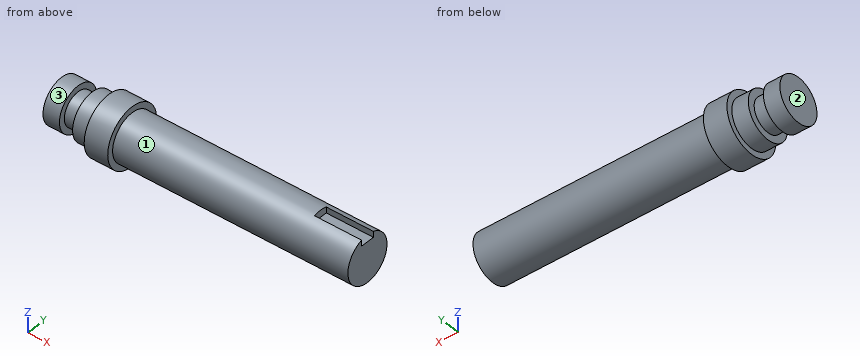
```python
from build123d import *

# Parameters (mm, degrees)
CUT_EXTRUDE1_DEPTH = 20


with BuildPart() as part:
    # Sketch1 → Revolve1 (revolve)
    with BuildSketch(Plane.XY, mode=Mode.PRIVATE) as revolve1_sk:
        Polygon((0, 0), (0, 9.5), (7, 9.5), (7, 7), (13, 7), (13, 10), (20, 10), (20, 12.5), (30, 12.5), (30, 10), (130, 10), (130, 0), align=None)
    revolve(revolve1_sk.sketch.rotate(Axis((130, 0, 0), (-1, 0, 0)), 90), axis=Axis((130, 0, 0), (-1, 0, 0)))

    # Sketch2 → Cut-Extrude1 (cut)
    with BuildSketch(Plane(origin=(130, 0, 0), x_dir=(0, 0, -1), z_dir=(1, 0, 0))):
        with BuildLine():
            Line((-9.539392014, 3), (-7.039392014, 3))
            Line((-7.039392014, 3), (-7.039392014, -3))
            Line((-7.039392014, -3), (-9.539392014, -3))
            ThreePointArc((-9.539392014, -3), (-10, 0), (-9.539392014, 3))
        make_face()
    extrude(amount=-CUT_EXTRUDE1_DEPTH, mode=Mode.SUBTRACT)


solid = part.part
```
The listing builds one solid part. Answer for the finished solid, in the listing's coordinates (mm). Face numbers are marked on the shaded views. A direction names the side the tool comes from. Round coordinates to 2 decimals unless told otherwise and drop trailing zeros. Loops run counter-clockwise (first coordinate to the right, second up) from the corner with the lowest first, then second, coordinate; pieces in that order, holes last.
Q1. Which of the six approach directions +Z, -Z, +X, -X, +Y, -Y give full straight-line access (tool end or side, diameter ignored) to the marked faces 1, 2 and 3?
Q2. Section C-C, the plane x = 56 is taken. Determine the outline of the cut face in (y, z), then the cut area to 3 significant figures.
Q3. Section A-A, the plane y = 0 is taken. Determine the outline of the cut face in (x, z).
Q4. Find the intervals of material crossed by line 1 (X direction, y = -2.5, z = 8.5); line 2 (X direction, y = -8.5, z = 1.5); line 3 (X direction, y = -11.5, z = 2.75), in increasing order.
Q5. Section B-B, the plane z = 0 is taken. Determine the outline of the cut face in (x, y).
Q6. Given pin 1 Ø6.5 at (x, y) = (124.5, -0.5) entering from +Z; pin 2 Ø6 at (x, z) = (31, -5.5) entering from -Y; pin 3 Ø6 at (x, y) = (74.5, -1) entering from -Z, each flat-ended and moving along its own axis, determine where each tip first touches the part or whether it passes through.
Completed:
1. face 1: +X
1. face 2: +Z, -Z, -X, +Y, -Y
1. face 3: -X
2. outline: circle Ø20 at (0, 0)
2. area: 314 mm2
3. outline: (0, -9.5) - (7, -9.5) - (7, -7) - (13, -7) - (13, -10) - (20, -10) - (20, -12.5) - (30, -12.5) - (30, -10) - (130, -10) - (130, 7.04) - (110, 7.04) - (110, 10) - (30, 10) - (30, 12.5) - (20, 12.5) - (20, 10) - (13, 10) - (13, 7) - (7, 7) - (7, 9.5) - (0, 9.5) - close
4. line 1: x = 0 to 7, 13 to 110
4. line 2: x = 0 to 7, 13 to 130
4. line 3: x = 20 to 30
5. outline: (0, -9.5) - (7, -9.5) - (7, -7) - (13, -7) - (13, -10) - (20, -10) - (20, -12.5) - (30, -12.5) - (30, -10) - (130, -10) - (130, 10) - (30, 10) - (30, 12.5) - (20, 12.5) - (20, 10) - (13, 10) - (13, 7) - (7, 7) - (7, 9.5) - (0, 9.5) - close
6. pin 1: stops at z = 9.54
6. pin 2: stops at y = -12.21
6. pin 3: stops at z = -10
